```python
from build123d import *

# Parameters (mm, degrees)
BOSS_EXTRUDE1_DEPTH             = 20
SKETCH6_W                       = 25
SKETCH6_H                       = 20
BOSS_EXTRUDE5_DEPTH             = 5.5
BOSS_EXTRUDE11_START            = -20
BOSS_EXTRUDE11_DEPTH            = 34
SKETCH4_R                       = 2
CUT_EXTRUDE1_DEPTH              = 10
BOSS_EXTRUDE13_DEPTH            = 12
FILLET11_START                  = 14.0499999
FILLET11_DEPTH                  = 7.9500001
FILLET11_START_2                = -14.996842371
FILLET11_2_DEPTH                = 30.996842371
SKETCH22_R                      = 2
CUT_EXTRUDE6_DEPTH              = 10
CHAMFER1_SIZE                   = 14
SKETCH26_W                      = 22
SKETCH26_H                      = 20
BOSS_EXTRUDE14_DEPTH            = 11
CUT_EXTRUDE7_DEPTH              = 2.5
CUT_EXTRUDE8_REACH              = 65.92
SKETCH27_R                      = 4
SKETCH27_R_2                    = 1.15
SKETCH27_R_3                    = 1.6
CUT_EXTRUDE9_DEPTH              = 2.5
BOSS_EXTRUDE15_DEPTH            = 1
BOSS_EXTRUDE15_DEPTH_BACK       = 2
SKETCH31_R                      = 4
SKETCH31_R_2                    = 1.65
SKETCH32_R                      = 2.85
SKETCH32_R_2                    = 2.25
CUT_EXTRUDE12_DEPTH             = 7
CUT_EXTRUDE12_DIRECTION_2_REACH = 61.046
SKETCH33_R                      = 3.8
BOSS_EXTRUDE17_DEPTH            = 7
FILLET17_R                      = 1
CUT_EXTRUDE13_DEPTH             = 14
SKETCH36_R                      = 2
CUT_EXTRUDE14_DEPTH             = 10
FILLET18_R                      = 10
CUT_EXTRUDE16_REACH             = 67.49
SKETCH37_W                      = 5.717933373
SKETCH37_H                      = 6
CHAMFER2_SIZE                   = 7
SKETCH38_W                      = 10
SKETCH38_H                      = 20
CUT_EXTRUDE17_DEPTH             = 4
CUT_EXTRUDE19_REACH             = 59.527
SKETCH39_W                      = 10
SKETCH39_H                      = 5
CUT_EXTRUDE20_DEPTH             = 83.61561247
CUT_EXTRUDE20_DEPTH_BACK        = 83.61561247
SKETCH40_W                      = 71.015717368
SKETCH40_H                      = 42.367018064


with BuildPart() as part:
    # Sketch1 → Boss-Extrude1 (new body)
    with BuildSketch(Plane(origin=(0, 0, 0), x_dir=(1, 0, 0), z_dir=(0, 1, 0))):
        Polygon((-15.5, -37), (-10, -37), (-10, 4), (11, 4), (11, -37), (18, -37), (18, -27), (21, -19), (21, 10), (-15.5, 10), align=None)
    extrude(amount=BOSS_EXTRUDE1_DEPTH)

    # Sketch6 → Boss-Extrude5 (add)
    with BuildSketch(Plane.ZY.offset(15.5)):
        with Locations((2.5, 10)):
            Rectangle(SKETCH6_W, SKETCH6_H)
    extrude(amount=BOSS_EXTRUDE5_DEPTH)

    # Sketch20 → Boss-Extrude11 (add)
    with BuildSketch(Plane(origin=(0, 20, 0), x_dir=(1, 0, 0), z_dir=(0, 1, 0)).offset(BOSS_EXTRUDE11_START)):
        Polygon((-21, 6.554166441), (14, 6.554166441), (14, -16.445833559), (21.006315459, -12.400735443), (21.006315459, 10.282066627), (15.003157729, 18.901571597), (-14.996842271, 18.901571597), (-21, 10.282066627), align=None)
    extrude(amount=BOSS_EXTRUDE11_DEPTH)

    # Sketch4 → Cut-Extrude1 (cut)
    with BuildSketch(Plane(origin=(0, 20, 0), x_dir=(1, 0, 0), z_dir=(0, 1, 0))):
        with Locations(Location((-4.375, 8, 0), (0, 0, 270))):
            Circle(SKETCH4_R)
        with Locations(Location((5.375, 8, 0), (0, 0, 270))):
            Circle(SKETCH4_R)
    extrude(amount=-CUT_EXTRUDE1_DEPTH, mode=Mode.SUBTRACT)

    # Sketch24 → Boss-Extrude13 (add)
    with BuildSketch(Plane(origin=(0, 34, 0), x_dir=(1, 0, 0), z_dir=(0, 1, 0))):
        with BuildLine():
            Line((-14.996842271, 18.901571597), (-14.420936492, 19.728473528))
            ThreePointArc((-14.420936492, 19.728473528), (-3.81756267, 26.467738085), (8.613124034, 24.643662635))
            ThreePointArc((8.613124034, 24.643662635), (12.140366622, 22.142331504), (15.003157729, 18.901571597))
            Line((15.003157729, 18.901571597), (21.006315459, 10.282066627))
            Line((21.006315459, 10.282066627), (21.006315459, 6.554166441))
            Line((21.006315459, 6.554166441), (-21, 6.554166441))
            Line((-21, 6.554166441), (-21, 10.282066627))
            Line((-21, 10.282066627), (-14.996842271, 18.901571597))
        make_face()
    extrude(amount=-BOSS_EXTRUDE13_DEPTH)

    # Fillet11: read off the stored shape, not the designer's step
    # Fillet11 outline → Fillet11 (add)
    with BuildSketch(Plane(origin=(0, 0, 0), x_dir=(1, 0, 0), z_dir=(0, 1, 0)).offset(FILLET11_START)):
        with BuildLine():
            Line((-14.996842271, 18.901571597), (15.003161757, 18.901565813))
            ThreePointArc((15.003161757, 18.901565813), (12.140369243, 22.142329149), (8.613124034, 24.643662635))
            ThreePointArc((8.613124034, 24.643662635), (-3.81756267, 26.467738085), (-14.420936492, 19.728473528))
            Line((-14.420936492, 19.728473528), (-14.996842271, 18.901571597))
        make_face()
    extrude(amount=FILLET11_DEPTH)

    # Fillet11 2 outline → Fillet11 2 (cut)
    with BuildSketch(Plane.YZ.offset(FILLET11_START_2)):
        with BuildLine():
            Line((22, -28), (22, -26.851571597))
            ThreePointArc((22, -26.851571597), (19.67149891, -21.230072687), (14.05, -18.901571597))
            Line((14.05, -18.901571597), (14.0499999, -28))
            Line((14.0499999, -28), (22, -28))
        make_face()
    extrude(amount=FILLET11_2_DEPTH, mode=Mode.SUBTRACT)

    # Sketch22 → Cut-Extrude6 (cut)
    with BuildSketch(Plane(origin=(0, 34, 0), x_dir=(1, 0, 0), z_dir=(0, 1, 0))):
        with Locations(Location((-14.720302421, 13.351367671, 0), (0, 0, 270))):
            Circle(SKETCH22_R)
        with Locations(Location((-3.067324575, 22.581252689, 0), (0, 0, 270))):
            Circle(SKETCH22_R)
    extrude(amount=-CUT_EXTRUDE6_DEPTH, mode=Mode.SUBTRACT)

    # Chamfer1
    chamfer1_edges = [part.edges().sort_by_distance(p)[0] for p in [
        (17.503157729, 34, 14.423284501),
    ]]
    chamfer(chamfer1_edges, length=CHAMFER1_SIZE)

    # Sketch26 → Boss-Extrude14 (add)
    with BuildSketch(Plane.ZY.offset(21)):
        with Locations((26, 10)):
            Rectangle(SKETCH26_W, SKETCH26_H)
    extrude(amount=-BOSS_EXTRUDE14_DEPTH)

    # Sketch25 → Cut-Extrude7 (cut)
    with BuildSketch(Plane.ZY.offset(21)):
        with BuildLine():
            Line((11.868890963, 14.931194411), (31.150048263, 18.330982662))
            ThreePointArc((31.150048263, 18.330982662), (35.639064994, 15.187739308), (32.49582164, 10.698722576))
            Line((32.49582164, 10.698722576), (13.21466434, 7.298934325))
            ThreePointArc((13.21466434, 7.298934325), (-1.168124774, 8.697638667), (11.868890963, 14.931194411))
        make_face()
    extrude(amount=-CUT_EXTRUDE7_DEPTH, mode=Mode.SUBTRACT)

    # Sketch27 → Cut-Extrude8 (cut, up to next)
    with BuildSketch(Plane.ZY.offset(18.5), mode=Mode.PRIVATE) as cut_extrude8_sk1:
        with Locations((6.217933373, 10)):
            Circle(SKETCH27_R)
    cut_extrude8_tool1 = extrude(cut_extrude8_sk1.sketch, amount=-CUT_EXTRUDE8_REACH, mode=Mode.PRIVATE) & part.part
    # Sketch27 → Cut-Extrude8 (cut, up to next)
    with BuildSketch(Plane.ZY.offset(18.5), mode=Mode.PRIVATE) as cut_extrude8_sk2:
        with Locations((15.08120315, 11.562833599)):
            Circle(SKETCH27_R_2)
    cut_extrude8_tool2 = extrude(cut_extrude8_sk2.sketch, amount=-CUT_EXTRUDE8_REACH, mode=Mode.PRIVATE) & part.part
    # Sketch27 → Cut-Extrude8 (cut, up to next)
    with BuildSketch(Plane.ZY.offset(18.5), mode=Mode.PRIVATE) as cut_extrude8_sk3:
        with Locations((27.883703939, 13.820259909)):
            Circle(SKETCH27_R_3)
    cut_extrude8_tool3 = extrude(cut_extrude8_sk3.sketch, amount=-CUT_EXTRUDE8_REACH, mode=Mode.PRIVATE) & part.part
    add(cut_extrude8_tool1.solids().sort_by_distance((-18.5, 10, 6.217933))[0], mode=Mode.SUBTRACT)
    add(cut_extrude8_tool2.solids().sort_by_distance((-18.5, 11.562834, 15.081203))[0], mode=Mode.SUBTRACT)
    add(cut_extrude8_tool3.solids().sort_by_distance((-18.5, 13.82026, 27.883704))[0], mode=Mode.SUBTRACT)

    # Sketch28 → Cut-Extrude9 (cut)
    with BuildSketch(Plane.ZY.offset(21)):
        Polygon((-0.028318142, 0.777915528), (-3.197748963, 15.950413947), (10.506443157, 18.813125656), (17.248705835, 15.879800924), (18.680061689, 9.027704864), (13.675873978, 3.640627238), align=None)
    extrude(amount=-CUT_EXTRUDE9_DEPTH, mode=Mode.SUBTRACT)

    # Sketch31 → Boss-Extrude15 (add, two sides: drawn at the far end of the back side and taken through both)
    with BuildSketch(Plane.ZY.offset(18.5).offset(-BOSS_EXTRUDE15_DEPTH_BACK)):
        with Locations((6.217933373, 10)):
            Circle(SKETCH31_R)
        with Locations((6.217933373, 10)):
            Circle(SKETCH31_R_2, mode=Mode.SUBTRACT)
    extrude(amount=BOSS_EXTRUDE15_DEPTH + BOSS_EXTRUDE15_DEPTH_BACK)

    # Sketch32 → Cut-Extrude12 (cut)
    with BuildSketch(Plane(origin=(-10, 0, 0), x_dir=(0, 0, -1), z_dir=(1, 0, 0))):
        with Locations((-27.883703939, 13.820259909)):
            Circle(SKETCH32_R)
        with Locations((-15.08120315, 11.562833599)):
            Circle(SKETCH32_R_2)
    extrude(amount=-CUT_EXTRUDE12_DEPTH, mode=Mode.SUBTRACT)

    # Sketch32 → Cut-Extrude12 direction 2 (cut, up to next)
    with BuildSketch(Plane(origin=(-10, 0, 0), x_dir=(0, 0, -1), z_dir=(1, 0, 0)), mode=Mode.PRIVATE) as cut_extrude12_direction_2_sk1:
        with Locations((-27.883703939, 13.820259909)):
            Circle(SKETCH32_R)
    cut_extrude12_direction_2_tool1 = extrude(cut_extrude12_direction_2_sk1.sketch, amount=CUT_EXTRUDE12_DIRECTION_2_REACH, mode=Mode.PRIVATE) & part.part
    # Sketch32 → Cut-Extrude12 direction 2 (cut, up to next)
    with BuildSketch(Plane(origin=(-10, 0, 0), x_dir=(0, 0, -1), z_dir=(1, 0, 0)), mode=Mode.PRIVATE) as cut_extrude12_direction_2_sk2:
        with Locations((-15.08120315, 11.562833599)):
            Circle(SKETCH32_R_2)
    cut_extrude12_direction_2_tool2 = extrude(cut_extrude12_direction_2_sk2.sketch, amount=CUT_EXTRUDE12_DIRECTION_2_REACH, mode=Mode.PRIVATE) & part.part
    add(cut_extrude12_direction_2_tool1.solids().sort_by_distance((-10, 13.82026, 27.883704))[0], mode=Mode.SUBTRACT)
    add(cut_extrude12_direction_2_tool2.solids().sort_by_distance((-10, 11.562834, 15.081203))[0], mode=Mode.SUBTRACT)

    # Sketch33 → Boss-Extrude17 (add)
    with BuildSketch(Plane(origin=(21.006315459, 0, 0), x_dir=(0, 0, -1), z_dir=(1, 0, 0))):
        with Locations((-6.217933373, 10)):
            Circle(SKETCH33_R)
    extrude(amount=BOSS_EXTRUDE17_DEPTH)

    # Fillet17
    fillet17_edges = [part.edges().sort_by_distance(p)[0] for p in [
        (28.006315459, 10, 10.017933373),
    ]]
    fillet(fillet17_edges, radius=FILLET17_R)

    # Sketch35 → Cut-Extrude13 (cut)
    with BuildSketch(Plane(origin=(0, 34, 0), x_dir=(1, 0, 0), z_dir=(0, 1, 0))):
        with BuildLine():
            Line((-19.79995418, 6.554166441), (14, 6.554166441))
            Line((14, 6.554166441), (14, 12.554166441))
            Line((14, 12.554166441), (-9.802737675, 12.554166441))
            ThreePointArc((-9.802737675, 12.554166441), (-11.071315957, 11.28171537), (-12.284990593, 9.956794065))
            ThreePointArc((-12.284990593, 9.956794065), (-15.675255632, 7.444453939), (-19.79995418, 6.554166441))
        make_face()
    extrude(amount=-CUT_EXTRUDE13_DEPTH, mode=Mode.SUBTRACT)

    # Sketch36 → Cut-Extrude14 (cut)
    with BuildSketch(Plane.XY.offset(37)):
        with Locations((-15.25, 14)):
            Circle(SKETCH36_R)
        with Locations((14.5, 10)):
            Circle(SKETCH36_R)
        with Locations((-15.25, 4)):
            Circle(SKETCH36_R)
    extrude(amount=-CUT_EXTRUDE14_DEPTH, mode=Mode.SUBTRACT)

    # Fillet18
    fillet18_edges = [part.edges().sort_by_distance(p)[0] for p in [
        (0.003157729, 0, -18.901571597),
    ]]
    fillet(fillet18_edges, radius=FILLET18_R)

    # Sketch37 → Cut-Extrude16 (cut, up to next)
    with BuildSketch(Plane(origin=(21, 0, 0), x_dir=(0, 0, -1), z_dir=(1, 0, 0)), mode=Mode.PRIVATE) as cut_extrude16_sk1:
        with Locations((1.141033313, 10)):
            Rectangle(SKETCH37_W, SKETCH37_H)
    cut_extrude16_tool1 = extrude(cut_extrude16_sk1.sketch, amount=-CUT_EXTRUDE16_REACH, mode=Mode.PRIVATE) & part.part
    add(cut_extrude16_tool1.solids().sort_by_distance((21, 10, -1.141033))[0], mode=Mode.SUBTRACT)

    # Chamfer2
    chamfer2_edges = [part.edges().sort_by_distance(p)[0] for p in [
        (11, 10, 1.717933373),
    ]]
    chamfer(chamfer2_edges, length=CHAMFER2_SIZE)

    # Sketch38 → Cut-Extrude17 (cut)
    with BuildSketch(Plane.XZ):
        with Locations((0.5, -14)):
            Rectangle(SKETCH38_W, SKETCH38_H)
    extrude(amount=-CUT_EXTRUDE17_DEPTH, mode=Mode.SUBTRACT)

    # Sketch39 → Cut-Extrude19 (cut, up to next)
    with BuildSketch(Plane(origin=(0, 34, 0), x_dir=(1, 0, 0), z_dir=(0, 1, 0)), mode=Mode.PRIVATE) as cut_extrude19_sk1:
        with Locations((0.5, 15.054166441)):
            Rectangle(SKETCH39_W, SKETCH39_H)
    cut_extrude19_tool1 = extrude(cut_extrude19_sk1.sketch, amount=-CUT_EXTRUDE19_REACH, mode=Mode.PRIVATE) & part.part
    add(cut_extrude19_tool1.solids().sort_by_distance((0.5, 34, -15.054166))[0], mode=Mode.SUBTRACT)


with BuildPart() as body_2:
    # Mirror1: mirrored copy
    add(part.part.mirror(Plane(origin=(0, -10, 0), x_dir=(0, 0, 1), z_dir=(0, -1, 0))))


with BuildPart() as part_1:
    add(part.part)

    # Sketch40 → Cut-Extrude20 (cut, two sides: drawn at the far end of the back side and taken through both)
    with BuildSketch(Plane(origin=(0, 0, -18.901571597), x_dir=(-1, 0, 0), z_dir=(0, 0, -1)).offset(-CUT_EXTRUDE20_DEPTH_BACK)):
        with Locations((-4.991813068, 18.312991293)):
            Rectangle(SKETCH40_W, SKETCH40_H)
    extrude(amount=CUT_EXTRUDE20_DEPTH + CUT_EXTRUDE20_DEPTH_BACK, mode=Mode.SUBTRACT)


solid = body_2.part
```
Geometry: final body of the model. Coordinates: model frame, mm. A direction names the side the tool comes from. Coordinates: 2 decimals unless noted, no trailing zeros. Order: outer loops, then holes, each group sorted by start corner. A loop starts at its lowest first (then second) coordinate and runs counter-clockwise, first axis right, second up. Notation, with made-up numbers: (65.5, 26.5) -> (86.5, 26.5) arc R14 ccw to (86.5, 43.5) -> close; hole circle Ø1 at (64.5, 82). An arc over 180 degrees is marked (long way). Write each question's results on one line, items separated by ' | '. Start each with the question number.
1) Mould query, pull axis Z, two halves, no side actions, for faces 6 (the flat face through (-19.768, -25.908, 15.782)), 7 (the flat face through (-15, -24, 27)), 8 (the flat face through (-21, -37.1, 15)), 9 (the cylindrical face through (5.46, -35.07, -10)). Classes: released by +Z, released by -Z, zero draft, split by the parting line, or undercut.
2) Set-up query: faces 1 (the cylindrical face through (-15.486, -49.07, -11.504)), 2 (the cylindrical face through (-13.451, -33.794, 15.374)), 3 (the flat face through (-19.768, -29.424, 25.266)), 4 (the cylindrical face through (14.066, -28.048, 32.07)), 5 (the flat face through (20, -30, 1.718)). Return all of +Z, -Z, +X, -X, +Y, -Y with unobstructed straight access to the full face (end or side cutting, diameter ignored); none if empty.
3) Cut plane D-D, the plane x = -8. Output: boundary loops of the cut face in (y, z), and give its area (3 significant figures).
4) Cut plane C-C, the plane z = -8. Output: boundary loops of the cut face in (x, y) (3 decimals).
5) Cut plane A-A, the plane x = 1.5. Output: boundary loops of the cut face in (y, z), and give its area (3 significant figures).
6) Cut plane B-B, the plane z = 22.5. Output: boundary loops of the cut face in (x, y).
7) Material intervals for line 1 along Z through (x, y) = (15, -33.5); line 2 along X through (y, z) = (-29.5, 13.5); line 3 along Z through (x, y) = (12.5, -34), sorted ascending.
8) First-contact query: pin 1 (4.5 mm diameter, centred on y = -33.82, z = 27.88, fed in from +X); pin 2 (2 mm diameter, centred on x = 10.5, y = -28, fed in from -Z); pin 3 (5 mm diameter, centred on y = -31.5, z = 15.5, fed in from +X); pin 4 (4 mm diameter, centred on y = -36.5, z = 6.5, fed in from -X). Flat tips, straight axial feed; report the tip coordinate or a pass-through.
Checks:
1) face 6: undercut | face 7: released by +Z | face 8: zero draft | face 9: undercut
2) face 1: -Y | face 2: +X | face 3: -X | face 4: +Z | face 5: none
3) outline: (-54, -25.02) -> (-41.79, -25.02) arc R7.95 cw to (-34.05, -18.9) -> (-30, -18.9) arc R10 ccw to (-20, -8.9) -> (-20, -4) -> (-40, -4) -> (-40, -12.55) -> (-54, -12.55) -> close | area: 452 mm^2
4) outline: (-21, -54) -> (-14.621, -54) -> (-14.621, -40) -> (-6.375, -40) -> (-6.375, -30) -> (-2.375, -30) -> (-2.375, -40) -> (3.375, -40) -> (3.375, -30) -> (7.375, -30) -> (7.375, -40) -> (14, -40) -> (14, -54) -> (21.006, -54) -> (21.006, -20) -> (5.5, -20) -> (5.5, -24) -> (-4.5, -24) -> (-4.5, -20) -> (-21, -20) -> close
5) outline: (-54, -26.8) -> (-42, -26.8) arc R7.95 cw to (-34.05, -18.9) -> (-30, -18.9) arc R10 ccw to (-24.99, -17.55) -> (-54, -17.55) -> close; (-40, -12.55) -> (-24, -12.55) -> (-24, -4) -> (-40, -4) -> close | area: 282 mm^2
6) outline: (-21, -40) -> (-10, -40) -> (-10, -20) -> (-21, -20) -> (-21, -28.94) -> (-18.5, -28.94) -> (-18.5, -36.81) -> (-21, -36.81) -> close; (11, -40) -> (19.69, -40) -> (19.69, -20) -> (11, -20) -> close
7) line 1: -18.9 to 13.94, 16.23 to 25.05, 30.72 to 37 | line 2: -18.5 to -10, 11 to 21 | line 3: -18.9 to 25.04, 30.73 to 37
8) pin 1: x = -17 | pin 2: z = -18.85 | pin 3: x = 21 | pin 4: x = -21
